Could you check a few things on this model? Use its own coordinates, in mm. A direction names the side the tool comes from. Round coordinates to 2 decimals unless told otherwise and drop trailing zeros. Loops run counter-clockwise (first coordinate to the right, second up) from the corner with the lowest first, then second, coordinate; pieces in that order, holes last. Notation, with made-up numbers: (77, 4) -> (101, 4) arc R14 ccw to (101, 31) -> close; hole circle Ø8 at (41, -27). An arc over 180 degrees is marked (long way). Put each result on its own line as item: value. Start each with the question number.
1. Imagine slicing it at B-B, the plane z = 19.05. Please give me the cut outline in (x, y), and give its area (3 significant figures).
2. I'm going to push flat-ended pins straight in: P1, Ø1.5, axis at x = 1, y = -13, coming from the -Z side; P2, Ø0.9, axis at x = 1.5, z = -18, coming from the -Y side; P3, Ø1.7, axis at y = -17.56, z = -6.35, coming from the +X side; P4, Ø1.5, axis at x = 2, y = -17.5, coming from the -Z side. Where does each tip first touch, or does it pass through?
3. Which directions (+Z, -Z, +X, -X, +Y, -Y) give clear straight access to the entire face, cutting with the end or side of a thin tool? Please do faces 1 (the flat face through (2, -18, 0)), 2 (the flat face through (2, -18, -12.7)), 3 (the flat face through (0, 0, 0)), 4 (the cylindrical face through (1.51, -0.55, -25.24)), 5 (the flat face through (2, 6.35, -24)).
4. Imagine slicing it at C-C, the plane x = 1.95. Count the separate pieces of the cut face and the enclosed holes in it, and give its area (3 significant figures).
5. I need wall thicknesses on line 1 (Z direction, x = 1.05, y = -12.5); line 2 (Z direction, x = 0.3, y = 10); line 3 (Y direction, x = 1.2, z = -16.5). Which ranges of each line are inside material? Lowest first, please. Write a range as [from, to].
6. Imagine slicing it at D-D, the plane y = -11. Please give me the cut outline in (x, z), and give its area (3 significant figures).
7. Imagine slicing it at A-A, the plane y = 0. Please give me the cut outline in (x, z).
8. If we mould it in two halves opening along Y, with no side actions, what happens to faces 6 (the cylindrical face through (1.507, -16.354, 18.278)), 7 (the flat face through (2.972, 0, 0)), 8 (the flat face through (1, 19.05, 8))? For each: pulls with the +Y half, pulls with the -Y half, needs draft (parallel to the pull), parting line crosses it, or undercut.
Autodesk Inventor part; units mm, degrees
ref_plane "YZ Plane" through (0, 0, 0) normal (1, 0, 0) x (0, 1, 0)
ref_plane "XZ Plane" through (0, 0, 0) normal (0, 1, 0) x (-1, 0, 0)
ref_plane "XY Plane" through (0, 0, 0) normal (0, 0, 1) x (1, 0, 0)
sketch "Sketch1" plane through (0, 0, 0) normal (1, 0, 0) x (0, 1, 0)
  line L0 (-19.05, 25.4) -> (19.05, 25.4)
  line L1 (19.05, 25.4) -> (19.05, -25.4)
  line L2 (19.05, -25.4) -> (-19.05, -25.4)
  line L3 (-19.05, -25.4) -> (-19.05, 25.4)
  line L4 (-19.05, 25.4) -> (19.05, -25.4) construction
  line L5 (19.05, 25.4) -> (-19.05, -25.4) construction
  point P0 (0, 0)
  dimension "d0" = 38.1
  dimension "d1" = 50.8
extrude "Extrusion1" add sketch "Sketch1" along normal blind 2.9718
sketch "Sketch2" plane through (2.9718, 0, 0) normal (1, 0, 0) x (0, 0, -1)
  line L0 (-25.4, -19.05) -> (25.4, -19.05)
  line L1 (25.4, -19.05) -> (12.7, -19.05)
  line L2 (12.7, -19.05) -> (12.7, -16.0782)
  line L3 (12.7, -16.0782) -> (25.4, -16.0782)
  line L4 (25.4, -16.0782) -> (25.4, -19.05)
  line L5 (0, -19.05) -> (-12.7, -19.05)
  line L6 (-12.7, -19.05) -> (-12.7, -16.0782)
  line L7 (-12.7, -16.0782) -> (0, -16.0782)
  line L8 (0, -16.0782) -> (0, -19.05)
  point P0 (0, 0)
  dimension "d4" = 12.7
  dimension "d5" = 2.9718
  dimension "d6" = 12.7
extrude "Extrusion2" cut sketch "Sketch2" against normal blind 2.9718
sketch "Sketch3" plane through (2.9718, 0, 0) normal (1, 0, 0) x (0, 0, -1)
  line L0 (25.4, -19.05) -> (22.4282, -19.05)
  line L1 (22.4282, -19.05) -> (22.4282, -6.35)
  line L2 (22.4282, -6.35) -> (25.4, -6.35)
  line L3 (25.4, -6.35) -> (25.4, -19.05)
  line L4 (0, -19.05) -> (12.7, -19.05)
  line L5 (25.4, -16.0782) -> (25.4, 19.05)
  line L6 (25.4, 6.35) -> (22.4282, 6.35)
  line L7 (22.4282, 6.35) -> (22.4282, 19.05)
  line L8 (22.4282, 19.05) -> (25.4, 19.05)
  line L9 (25.4, 19.05) -> (25.4, 6.35)
  point P0 (0, 0)
  point P1 (25.4, 9.3218)
  dimension "d9" = 0
  dimension "d10" = 0
  dimension "d11" = 12.7
  dimension "d12" = 2.9718
  dimension "d15" = 25.4
extrude "Extrusion3" cut sketch "Sketch3" against normal blind 25.4
fillet "Fillet1" radius 12.7 1 edges at (1.4859, 19.05, -22.4282)
sketch "Sketch4" plane through (2.9718, 0, 0) normal (1, 0, 0) x (0, 0, -1)
  circle A0 centre (23.9141, 0) radius 1.4351
  line L0 (25.4, -6.35) -> (25.4, 6.35)
  circle A1 centre (6.35, -17.5641) radius 1.4351
  circle A2 centre (-19.05, -17.5641) radius 1.4351
  line L1 (22.4282, -6.35) -> (25.4, -6.35)
  line L2 (12.7, -19.05) -> (12.7, -16.0782)
  line L3 (0, -19.05) -> (12.7, -19.05)
  line L4 (-25.4, -19.05) -> (-12.7, -19.05)
  line L5 (-12.7, -19.05) -> (-12.7, -16.0782)
  point P0 (0, 0)
  dimension "d23" = 2.8702
  dimension "d24" = 1.4859
  dimension "d25" = 2.8702
  dimension "d26" = 2.8702
  dimension "d27" = 6.35
  dimension "d28" = 6.35
  dimension "d29" = 1.4859
  dimension "d30" = 1.4859
  dimension "d31" = 6.35
extrude "Extrusion4" cut sketch "Sketch4" against normal blind 25.4
properties part number "side1"
Entries:
1. outline: (0, -19.05) -> (2.97, -19.05) -> (2.97, -19) -> (0, -19) -> close; (0, -16.13) -> (2.97, -16.13) -> (2.97, 19.05) -> (0, 19.05) -> close
1. area: 105 mm^2
2. P1: z = -22.43
2. P2: y = -16.08
2. P3: through
2. P4: z = -12.7
3. face 1: +X, -X, -Y
3. face 2: -Z, +X, -X, -Y
3. face 3: +Z, -Z, -X, +Y, -Y
3. face 4: +X, -X
3. face 5: -Z, +X, -X, +Y
4. separate pieces: 1
4. enclosed holes: 3
4. area: 1,740 mm^2
5. line 1: [-22.43, 25.4]
5. line 2: [-21.89, 25.4]
5. line 3: [-16.08, 17.09]
6. outline: (0, -22.43) -> (2.97, -22.43) -> (2.97, 25.4) -> (0, 25.4) -> close
6. area: 142 mm^2
7. outline: (0, -25.4) -> (2.97, -25.4) -> (2.97, -25.35) -> (0, -25.35) -> close; (0, -22.48) -> (2.97, -22.48) -> (2.97, 25.4) -> (0, 25.4) -> close
8. face 6: undercut
8. face 7: needs draft
8. face 8: pulls with the +Y half
